Can you work these out from the model? Positions are in its coordinate system, mm. A direction names the side the tool comes from. Give positions to 0.01 mm unless a question says otherwise; leave off trailing zeros. Loops run counter-clockwise (first coordinate to the right, second up) from the corner with the lowest first, then second, coordinate; pieces in that order, holes last. Notation, with made-up numbers: (40.5, 67) - (53.5, 67) arc R12 cw to (53.5, 82) - close; hole circle Ø10 at (89, -30.5). An arc over 180 degrees is marked (long way). Answer in a Markdown table with one row per item.
from build123d import *

# Parameters (mm, degrees)
SKETCH1_W                = 50
SKETCH1_H                = 3
BOSS_EXTRUDE1_DEPTH      = 50
SKETCH2_R                = 5
BOSS_EXTRUDE2_DEPTH      = 14.5
BOSS_EXTRUDE2_DEPTH_BACK = 14.5
SKETCH3_R                = 2.25
BOSS_EXTRUDE3_DEPTH      = 2
FILLET2_R                = 1
FILLET2_OF_MIRROR1_R     = 1
CUT_EXTRUDE1_DEPTH       = 11.5


with BuildPart() as part:
    # Sketch1 → Boss-Extrude1 (new body)
    with BuildSketch(Plane(origin=(0, 0, 0), x_dir=(1, 0, 0), z_dir=(0, 1, 0))):
        Rectangle(SKETCH1_W, SKETCH1_H)
    extrude(amount=BOSS_EXTRUDE1_DEPTH)

    # Sketch2 → Boss-Extrude2 (add, two sides)
    with BuildSketch(Plane(origin=(0, 0, 0), x_dir=(0, 0, -1), z_dir=(1, 0, 0))) as boss_extrude2_sk:
        with Locations((2.940369627, 52.589467232)):
            Circle(SKETCH2_R)
    extrude(amount=BOSS_EXTRUDE2_DEPTH)
    extrude(boss_extrude2_sk.sketch, amount=-BOSS_EXTRUDE2_DEPTH_BACK)

    # Sketch3 → Boss-Extrude3 (add)
    with BuildSketch(Plane(origin=(14.5, 0, 0), x_dir=(0, 0, -1), z_dir=(1, 0, 0))):
        with Locations((2.940369627, 52.589467232)):
            Circle(SKETCH3_R)
    boss_extrude3 = extrude(amount=BOSS_EXTRUDE3_DEPTH)

    # Fillet2
    fillet2_edges = [part.edges().sort_by_distance(p)[0] for p in [
        (16.5, 52.589467232, -0.690369627),
    ]]
    fillet(fillet2_edges, radius=FILLET2_R)

    # Mirror1: Boss-Extrude3 across plane
    add(boss_extrude3.mirror(Plane(origin=(0, 0, 0), x_dir=(0, 0, 1), z_dir=(1, 0, 0))))

    # Fillet2 of Mirror1
    fillet2_of_mirror1_edges = [part.edges().sort_by_distance(p)[0] for p in [
        (-16.5, 52.589467232, -0.690369627),
    ]]
    fillet(fillet2_of_mirror1_edges, radius=FILLET2_OF_MIRROR1_R)

    # Sketch4 → Cut-Extrude1 (cut, through all)
    with BuildSketch(Plane(origin=(14.5, 0, 0), x_dir=(0, 0, -1), z_dir=(1, 0, 0))):
        with BuildLine():
            Line((1.5, 50), (1.5, 47.801426366))
            ThreePointArc((1.5, 47.801426366), (-0.122497577, 48.637398851), (-1.336856045, 50))
            Line((-1.336856045, 50), (1.5, 50))
        make_face()
    cut_extrude1 = extrude(amount=CUT_EXTRUDE1_DEPTH, mode=Mode.SUBTRACT)

    # Mirror2: Cut-Extrude1 across plane
    add(cut_extrude1.mirror(Plane(origin=(0, 0, 0), x_dir=(0, 0, 1), z_dir=(1, 0, 0))), mode=Mode.SUBTRACT)


solid = part.part
Q1. Imagine slicing it at D-D, the plane z = -6.75. Write out the boundary of the cut face in (x, y).
Checked values:
| item | result |
|---|---|
| outline | (-14.5, 49.35) - (14.5, 49.35) - (14.5, 55.83) - (-14.5, 55.83) - close |
Q2. For pin 1 (15 mm diameter, centred on x = -12, y = 27, fed in from +Z); pin 2 (1.5 mm diameter, centred on x = -4.5, z = -6.5, fed in from +Y); pin 3 (0.8 mm diameter, centred on y = 53, z = -2.5, fed in from -X), each with a flat end and sliding along its axis, tell me the tip position at first contact or that it passes through.
Checked values:
| item | result |
|---|---|
| pin 1 | stops at z = 1.5 |
| pin 2 | stops at y = 56.73 |
| pin 3 | stops at x = -16.5 |
Q3. On a 3-axis mill with a long thin cutter (end or side, diameter ignored), from which of +Z, -Z, +X, -X, +Y, -Y can I reach the whole of each face in a straight line? I mean faces 1 (the face through (16.5, 53, -3)), 2 (the face through (14.5, 50, -4)), 3 (the face through (-14.99, 54.82, -2.65)), 4 (the face through (0, 25, 1.5)), 5 (the face through (-16.5, 53, -3)). Say none if no direction works.
Checked values:
| item | result |
|---|---|
| face 1 | +Z, -Z, +X, +Y, -Y |
| face 2 | +X |
| face 3 | -X |
| face 4 | +Z, +X, -X, -Y |
| face 5 | +Z, -Z, -X, +Y, -Y |
Q4. Imagine slicing it at C-C, the plane x = 18. Write out the boundary of the cut face in (y, z), and give its area (3 significant figures).
Checked values:
| item | result |
|---|---|
| outline | (0, -1.5) - (47.8, -1.5) arc R5 cw to (50, 1.34) - (50, 1.5) - (0, 1.5) - close |
| area | 146 mm² |
Q5. If I drill on line 1 (Z direction, x = 12, y = 36.5); line 2 (X direction, y = 53, z = -4); line 3 (X direction, y = 54, z = 1), over which ranges is the centre line in solid material (lowest first)? Write a range as [from, to].
Checked values:
| item | result |
|---|---|
| line 1 | z = [-1.5, 1.5] |
| line 2 | x = [-16.5, 16.5] |
| line 3 | x = [-14.5, 14.5] |
Q6. Imagine slicing it at B-B, the plane y = 26. Write out the boundary of the cut face in (x, z).
Checked values:
| item | result |
|---|---|
| outline | (-25, -1.5) - (25, -1.5) - (25, 1.5) - (-25, 1.5) - close |
Q7. Imagine slicing it at A-A, the plane x = -11. Write out the boundary of the cut face in (y, z).
Checked values:
| item | result |
|---|---|
| outline | (0, -1.5) - (47.8, -1.5) arc R5 ccw (long way) to (50, 1.34) - (50, 1.5) - (0, 1.5) - close |
